from build123d import *

# Parameters (mm, degrees)
SKETCH_1_W      = 15
SKETCH_1_H      = 5
EXTRUDE_1_DEPTH = 50
SKETCH_2_W      = 7.5
SKETCH_2_H      = 50
EXTRUDE_2_DEPTH = 12
SKETCH_3_W      = 50
SKETCH_3_H      = 12
EXTRUDE_3_DEPTH = 60
SKETCH_4_W      = 15
SKETCH_4_H      = 50
EXTRUDE_4_DEPTH = 5


with BuildPart() as part:
    # 스케치1 → 보스-돌출1 (new body)
    with BuildSketch(Plane.XY):
        with Locations((7.5, 2.5)):
            Rectangle(SKETCH_1_W, SKETCH_1_H)
    extrude(amount=EXTRUDE_1_DEPTH)

    # 스케치2 → 보스-돌출2 (add)
    with BuildSketch(Plane.XZ):
        with Locations((11.25, 25)):
            Rectangle(SKETCH_2_W, SKETCH_2_H)
    extrude(amount=EXTRUDE_2_DEPTH)

    # 스케치3 → 보스-돌출3 (add)
    with BuildSketch(Plane(origin=(15, 0, 0), x_dir=(0, 0, -1), z_dir=(1, 0, 0))):
        with Locations((-25, -6)):
            Rectangle(SKETCH_3_W, SKETCH_3_H)
    extrude(amount=EXTRUDE_3_DEPTH)

    # 스케치4 → 보스-돌출4 (add)
    with BuildSketch(Plane(origin=(0, 0, 0), x_dir=(1, 0, 0), z_dir=(0, 1, 0))):
        with Locations((67.5, -25)):
            Rectangle(SKETCH_4_W, SKETCH_4_H)
    extrude(amount=EXTRUDE_4_DEPTH)


solid = part.part
Verification items for the finished model (mm, model axes). A direction names the side the tool comes from. Give positions to 0.01 mm unless a question says otherwise; leave off trailing zeros. Loops run counter-clockwise (first coordinate to the right, second up) from the corner with the lowest first, then second, coordinate; pieces in that order, holes last. Notation, with made-up numbers: (42.25, -3.5) - (65.25, -3.5) arc R19 cw to (65.25, 6.5) - close; hole circle Ø3 at (43.25, 11.5). An arc over 180 degrees is marked (long way). Write item = value, one per line. Start each with the question number.
Q1. Thickness scan on line 1 (X direction, y = 1.25, z = 3); line 2 (X direction, y = -4, z = 10); line 3 (Y direction, x = 42, z = 45). Record the ranges inside material, lowest first.
Q2. Mould release check, pull along X, two halves, no side actions. Record for faces 4 (the face through (60, 2, 25)), 5 (the face through (75, -4, 25)), 6 (the face through (37, -6, 0)): released by +X, released by -X, zero draft, split by the parting line, or undercut.
Q3. Tool access check on faces 1 (the face through (4, 0, 25)), 2 (the face through (67, 5, 25)), 3 (the face through (15, 3, 25)). Record the directions out of +Z, -Z, +X, -X, +Y, -Y that give a thin tool (end or side, any length) a straight path to the whole face; none if there is none.
Q4. Cross-section at B-B, the plane z = 19. Enter the section's corners in (x, y), and give its area (3 significant figures).
Q5. Cross-section at C-C, the plane x = 24.5. Enter the section's corners in (y, z).
Q6. Cross-section at A-A, the plane y = 1. Enter the section's corners in (x, z).
Q7. Depth check by flat-ended pin: P1, Ø4, axis at y = -4, z = 11.5, coming from the -X side; P2, Ø2, axis at x = 39.5, z = 25.5, coming from the +Y side; P3, Ø6, axis at x = 4, z = 15, coming from the -Y side. Enter the tip coordinate at first touch or a pass-through.
Answer key:
q1.line_1 = 0 to 15, 60 to 75
q1.line_2 = 7.5 to 75
q1.line_3 = -12 to 0
q2.face_4 = undercut
q2.face_5 = released by +X
q2.face_6 = zero draft
q3.face_1 = +Z, -Z, -X, -Y
q3.face_2 = +Z, -Z, +X, -X, +Y
q3.face_3 = +Z, -Z, +Y
q4.outline = (0, 0) - (7.5, 0) - (7.5, -12) - (75, -12) - (75, 5) - (60, 5) - (60, 0) - (15, 0) - (15, 5) - (0, 5) - close
q4.area = 960 mm^2
q5.outline = (-12, 0) - (0, 0) - (0, 50) - (-12, 50) - close
q6.outline = (0, 0) - (15, 0) - (15, 50) - (0, 50) - close; (60, 0) - (75, 0) - (75, 50) - (60, 50) - close
q7.P1 = 7.5
q7.P2 = 0
q7.P3 = 0
